```python
from build123d import *

# Parameters (mm, degrees)
F0_W     = 124.46
F0_H     = 2.54
F0_W_2   = 2.54
F0_H_2   = 414.02
F1_DEPTH = 5.08


with BuildPart() as f1:
    # F0 (on Front) → F1 (new body)
    with BuildSketch(Plane.XZ):
        with Locations((62.23, 1.27)):
            Rectangle(F0_W, F0_H)
        with Locations((125.73, 1.27)):
            Rectangle(F0_W_2, F0_H)
        with Locations((125.73, 209.55)):
            Rectangle(F0_W_2, F0_H_2)
        Polygon((-53.34, 416.56), (124.46, 416.56), (127, 416.56), (127, 419.1), (-53.34, 419.1), align=None)
    extrude(amount=F1_DEPTH)


solid = f1.part
```
For this review, take the finished solid that the model builds, in its own axes (mm). Round coordinates to 2 decimals unless told otherwise and drop trailing zeros. Order: outer loops, then holes, each group sorted by start corner. A loop starts at its lowest first (then second) coordinate and runs counter-clockwise, first axis right, second up.
Q1. Insertion check: P1, Ø0.8, axis at y = -2, z = 1.5, coming from the -X side; P2, Ø2.5, axis at y = -3, z = 222.5, coming from the -X side. Each pin has a flat end and moves straight along its axis. Give the tip position at first contact, or say it passes through.
Findings below:
P1: stops at x = 0
P2: stops at x = 124.46
Q2. We need section C-C, the plane x = -39.5. Give the boundary of the cut face in (y, z).
Findings below:
outline: (-5.08, 416.56) - (0, 416.56) - (0, 419.1) - (-5.08, 419.1) - close
Q3. We need section D-D, the plane z = 269.5. Give the boundary of the cut face in (x, y).
Findings below:
outline: (124.46, -5.08) - (127, -5.08) - (127, 0) - (124.46, 0) - close
Q4. Wall thickness on line 1 (Z direction, x = 11.5, y = -0.4); line 2 (Z direction, x = -15, y = -3.35); line 3 (X direction, y = -2.9, z = 249): over which ranges is each line inside the solid? List them lowest first.
Findings below:
line 1: z = 0 to 2.54, 416.56 to 419.1
line 2: z = 416.56 to 419.1
line 3: x = 124.46 to 127
Q5. We need section B-B, the plane y = -4.15. Give the boundary of the cut face in (x, z), plus the area to 3 significant figures.
Findings below:
outline: (-53.34, 416.56) - (124.46, 416.56) - (124.46, 2.54) - (0, 2.54) - (0, 0) - (127, 0) - (127, 419.1) - (-53.34, 419.1) - close
area: 1,830 mm2
Q6. We need section A-A, the plane x = 62. Give the boundary of the cut face in (y, z).
Findings below:
outline: (-5.08, 0) - (0, 0) - (0, 2.54) - (-5.08, 2.54) - close; (-5.08, 416.56) - (0, 416.56) - (0, 419.1) - (-5.08, 419.1) - close
